```python
from build123d import *

# Parameters (mm, degrees)
BOSS_EXTRUDE1_DEPTH            = 11.43
BOSS_EXTRUDE1_DEPTH_BACK       = 101.6
CUT_EXTRUDE2_REACH             = 833.724
CUT_EXTRUDE2_DIRECTION_2_REACH = 833.724
CUT_EXTRUDE3_REACH             = 833.724
CUT_EXTRUDE3_DIRECTION_2_REACH = 833.724
BOSS_EXTRUDE3_DEPTH            = 149.606
SKETCH9_R                      = 19.05
BOSS_EXTRUDE4_DEPTH            = 101.6
CUT_EXTRUDE4_REACH             = 936.966
CUT_EXTRUDE4_DIRECTION_2_REACH = 936.966
CUT_EXTRUDE5_REACH             = 936.966
CUT_EXTRUDE5_DIRECTION_2_REACH = 936.966


with BuildPart() as part:
    # Sketch1 → Boss-Extrude1 (new, two sides: drawn at the far end of the back side and taken through both)
    with BuildSketch(Plane.XY.offset(-BOSS_EXTRUDE1_DEPTH_BACK)):
        Polygon((-787.4, -209.55), (-787.471663752, -247.65), (-762.071663752, -247.65), (-762.071663752, -209.55), (-203.2, 215.9), (0, 215.9), (0, 241.3), (-203.2, 241.3), (-787.4, -207.01), align=None)
        Polygon((0, 241.3), (0, 215.9), (203.2, 215.9), (762.071663752, -209.55), (762.071663752, -247.65), (787.471663752, -247.65), (787.4, -209.55), (787.4, -207.01), (203.2, 241.3), align=None)
    extrude(amount=BOSS_EXTRUDE1_DEPTH + BOSS_EXTRUDE1_DEPTH_BACK)

    # Sketch5 → Cut-Extrude2 (cut, up to next)
    with BuildSketch(Plane(origin=(0, 0, 0), x_dir=(0, 0, -1), z_dir=(1, 0, 0)), mode=Mode.PRIVATE) as cut_extrude2_sk1:
        Polygon((-11.43, -209.55), (0, 215.9), (0, 241.3), (-11.43, 241.3), (-11.43, 215.9), align=None)
    cut_extrude2_tool1 = extrude(cut_extrude2_sk1.sketch, amount=-CUT_EXTRUDE2_REACH, mode=Mode.PRIVATE) & part.part
    add(cut_extrude2_tool1.solids().sort_by_distance((0, 90.565111, 7.4168))[0], mode=Mode.SUBTRACT)

    # Sketch5 → Cut-Extrude2 direction 2 (cut, up to next)
    with BuildSketch(Plane(origin=(0, 0, 0), x_dir=(0, 0, -1), z_dir=(1, 0, 0)), mode=Mode.PRIVATE) as cut_extrude2_direction_2_sk1:
        Polygon((-11.43, -209.55), (0, 215.9), (0, 241.3), (-11.43, 241.3), (-11.43, 215.9), align=None)
    cut_extrude2_direction_2_tool1 = extrude(cut_extrude2_direction_2_sk1.sketch, amount=CUT_EXTRUDE2_DIRECTION_2_REACH, mode=Mode.PRIVATE) & part.part
    add(cut_extrude2_direction_2_tool1.solids().sort_by_distance((0, 90.565111, 7.4168))[0], mode=Mode.SUBTRACT)

    # Sketch7 → Cut-Extrude3 (cut, up to next)
    with BuildSketch(Plane(origin=(0, 0, 0), x_dir=(0, 0, -1), z_dir=(1, 0, 0)), mode=Mode.PRIVATE) as cut_extrude3_sk1:
        Polygon((26.67, -209.55), (101.6, 223.982414479), (101.6, -247.65), (26.67, -247.65), align=None)
    cut_extrude3_tool1 = extrude(cut_extrude3_sk1.sketch, amount=-CUT_EXTRUDE3_REACH, mode=Mode.PRIVATE) & part.part
    add(cut_extrude3_tool1.solids().sort_by_distance((0, -89.489932, -74.75645))[0], mode=Mode.SUBTRACT)

    # Sketch7 → Cut-Extrude3 direction 2 (cut, up to next)
    with BuildSketch(Plane(origin=(0, 0, 0), x_dir=(0, 0, -1), z_dir=(1, 0, 0)), mode=Mode.PRIVATE) as cut_extrude3_direction_2_sk1:
        Polygon((26.67, -209.55), (101.6, 223.982414479), (101.6, -247.65), (26.67, -247.65), align=None)
    cut_extrude3_direction_2_tool1 = extrude(cut_extrude3_direction_2_sk1.sketch, amount=CUT_EXTRUDE3_DIRECTION_2_REACH, mode=Mode.PRIVATE) & part.part
    add(cut_extrude3_direction_2_tool1.solids().sort_by_distance((0, -89.489932, -74.75645))[0], mode=Mode.SUBTRACT)

    # Sketch8 → Boss-Extrude3 (add)
    with BuildSketch(Plane.XY):
        Polygon((-787.471663752, -247.65), (-762.071663752, -247.65), (-762.071663752, -209.55), (-203.2, 215.9), (203.2, 215.9), (762.071663752, -209.55), (762.071663752, -247.65), (787.471663752, -247.65), (787.4, -207.01), (203.2, 241.3), (-203.2, 241.3), (-787.4, -207.01), align=None)
    extrude(amount=BOSS_EXTRUDE3_DEPTH)

    # Sketch9 → Boss-Extrude4 (add)
    with BuildSketch(Plane(origin=(787.032515479, 1.387837182, 0), x_dir=(0, 0, -1), z_dir=(0.9999984452495948, 0.0017633769855495952, 0))):
        with Locations(Location((-130.556, -229.988224375, 0), (0, 0, 270))):
            Circle(SKETCH9_R)
    boss_extrude4 = extrude(amount=BOSS_EXTRUDE4_DEPTH)

    # Mirror1: Boss-Extrude4 across plane
    add(boss_extrude4.mirror(Plane(origin=(0, 0, 0), x_dir=(0, 0, 1), z_dir=(1, 0, 0))))

    # Cut-Extrude4: up to this face of the body (flat: up to its plane)
    cut_extrude4_end = Plane(part.part.faces().sort_by_distance((-477.863853052, 30.525347549, 40.754880745))[0])
    # Sketch10 → Cut-Extrude4 (cut, up to the picked face)
    with BuildSketch(Plane(origin=(0, 0, 0), x_dir=(0, 0, -1), z_dir=(1, 0, 0)), mode=Mode.PRIVATE) as cut_extrude4_sk1:
        Polygon((-111.506, -207.01), (-111.506, -247.65), (101.6, -247.65), (101.6, 215.9), align=None)
    cut_extrude4_tool1 = split(extrude(cut_extrude4_sk1.sketch, amount=-CUT_EXTRUDE4_REACH, mode=Mode.PRIVATE), bisect_by=cut_extrude4_end, keep=Keep.BOTH, mode=Mode.PRIVATE)
    add(cut_extrude4_tool1.solids().sort_by(Axis((0, -92.041411, -24.838897), (-1, 0, 0)))[0], mode=Mode.SUBTRACT)

    # Cut-Extrude4 direction 2: up to this face of the body (flat: up to its plane)
    cut_extrude4_direction_2_end = Plane(part.part.faces().sort_by_distance((477.863853052, 30.525347549, 40.754880745))[0])
    # Sketch10 → Cut-Extrude4 direction 2 (cut, up to the picked face)
    with BuildSketch(Plane(origin=(0, 0, 0), x_dir=(0, 0, -1), z_dir=(1, 0, 0)), mode=Mode.PRIVATE) as cut_extrude4_direction_2_sk1:
        Polygon((-111.506, -207.01), (-111.506, -247.65), (101.6, -247.65), (101.6, 215.9), align=None)
    cut_extrude4_direction_2_tool1 = split(extrude(cut_extrude4_direction_2_sk1.sketch, amount=CUT_EXTRUDE4_DIRECTION_2_REACH, mode=Mode.PRIVATE), bisect_by=cut_extrude4_direction_2_end, keep=Keep.BOTH, mode=Mode.PRIVATE)
    add(cut_extrude4_direction_2_tool1.solids().sort_by(Axis((0, -92.041411, -24.838897), (1, 0, 0)))[0], mode=Mode.SUBTRACT)

    # Cut-Extrude5: up to this plane
    cut_extrude5_end = Plane(origin=(-191.85340904, 250.007275237, 11.43), z_dir=(-0.6087935435147127, 0.7933286969313537, 0))
    # Sketch11 → Cut-Extrude5 (cut, up to the surface)
    with BuildSketch(Plane(origin=(0, 0, 0), x_dir=(0, 0, -1), z_dir=(1, 0, 0)), mode=Mode.PRIVATE) as cut_extrude5_sk1:
        Polygon((0, 241.3), (-149.606, 241.3), (-149.606, -207.01), (0, 215.9), align=None)
    cut_extrude5_tool1 = split(extrude(cut_extrude5_sk1.sketch, amount=-CUT_EXTRUDE5_REACH, mode=Mode.PRIVATE), bisect_by=cut_extrude5_end, keep=Keep.BOTH, mode=Mode.PRIVATE)
    add(cut_extrude5_tool1.solids().sort_by_distance((0, 91.409357, 97.06341))[0], mode=Mode.SUBTRACT)

    # Cut-Extrude5 direction 2: up to this plane
    cut_extrude5_direction_2_end = Plane(origin=(191.85340904, 250.007275237, 11.43), z_dir=(-0.608793543514713, -0.7933286969313534, 0))
    # Sketch11 → Cut-Extrude5 direction 2 (cut, up to the surface)
    with BuildSketch(Plane(origin=(0, 0, 0), x_dir=(0, 0, -1), z_dir=(1, 0, 0)), mode=Mode.PRIVATE) as cut_extrude5_direction_2_sk1:
        Polygon((0, 241.3), (-149.606, 241.3), (-149.606, -207.01), (0, 215.9), align=None)
    cut_extrude5_direction_2_tool1 = split(extrude(cut_extrude5_direction_2_sk1.sketch, amount=CUT_EXTRUDE5_DIRECTION_2_REACH, mode=Mode.PRIVATE), bisect_by=cut_extrude5_direction_2_end, keep=Keep.BOTH, mode=Mode.PRIVATE)
    add(cut_extrude5_direction_2_tool1.solids().sort_by_distance((0, 91.409357, 97.06341))[0], mode=Mode.SUBTRACT)


solid = part.part
```
Geometry check sheet. Reference: the model listing, model coordinates, mm. A direction names the side the tool comes from. Give positions to 0.01 mm unless a question says otherwise; leave off trailing zeros. Order: outer loops, then holes, each group sorted by start corner. A loop starts at its lowest first (then second) coordinate and runs counter-clockwise, first axis right, second up. Notation, with made-up numbers: (58, 0.25) - (71, 0.25) arc R15 cw to (71, 13.25) - close; hole circle Ø7 at (13, -23). An arc over 180 degrees is marked (long way). Write item = value, one per line. Start each with the question number.
1) Draft check along X on faces 3 (the flat face through (776, -227, 111.506)), 4 (the flat face through (453.4, 49.3, 14.1)), 5 (the flat face through (439.934, 35.683, 33.371)). Enter one of: released by +X, released by -X, zero draft, split by the parting line, or undercut.
2) Section check A-A (y = 184). Enter the section's corners in (x, z), then the cut area to 3 significant figures.
3) Section check B-B (z = 43). Enter the section's corners in (x, y), then the cut area to 3 significant figures.
4) Gauge pin test, flat ends, axial feed: pin 1 Ø14.5 at (x, y) = (779.5, -225) entering from -Z; pin 2 Ø1.5 at (y, z) = (178.5, -25) entering from -X; pin 3 Ø6 at (x, z) = (515.5, 74.5) entering from -Y; pin 4 Ø3 at (x, z) = (95, 3) entering from +Y. Record the tip position at first contact, or that the pin passes through.
5) Access from +Z, -Z, +X, -X, +Y, -Y to the whole of each face (thin tool, end or side, straight path). Record for faces 1 (the flat face through (-442.54, 33.7, 24.12)), 2 (the flat face through (-776, -227, 111.506)).
6) Scan lines: L1, parallel to Y at x = -20, z = -83; L2, parallel to X at y = -58.5, z = 45.5; L3, parallel to X at y = 181.5, z = -77. Record each from-to range of solid material in increasing order.
7) Section check D-D (z = -75.5). Enter the section's corners in (x, y).
8) Section check C-C (x = -29). Enter the section's corners in (y, z), then the cut area to 4 significant figures.
Geometry check:
q1.face_3 = zero draft
q1.face_4 = released by +X
q1.face_5 = undercut
q2.outline = (-277.87, -85.53) - (-245.1, -85.53) - (-245.1, 11.28) - (-277.87, 11.28) - close; (245.1, -85.53) - (277.87, -85.53) - (277.87, 11.28) - (245.1, 11.28) - close
q2.area = 6,340 mm2
q3.outline = (-610.24, -71.06) - (-580.15, -71.06) - (-362.87, 94.35) - (-394.7, 94.35) - close; (362.87, 94.35) - (580.15, -71.06) - (610.24, -71.06) - (394.7, 94.35) - close
q3.area = 10,200 mm2
q4.pin_1 = 111.51
q4.pin_2 = -286.01
q4.pin_3 = -24.13
q4.pin_4 = through
q5.face_1 = +Z, -Z, -Y
q5.face_2 = -Z, +X, -X, -Y
q6.L1 = 215.9 to 241.3
q6.L2 = -593.87 to -563.65, 563.65 to 593.87
q6.L3 = -281.13 to -248.39, 248.39 to 281.13
q7.outline = (-303.79, 164.1) - (-271.24, 164.1) - (-203.2, 215.9) - (203.2, 215.9) - (271.24, 164.1) - (303.79, 164.1) - (203.2, 241.3) - (-203.2, 241.3) - close
q8.outline = (215.9, -100.2) - (223.98, -101.6) - (241.3, -101.6) - (241.3, 0) - (215.9, 0) - close
q8.area = 2,575 mm2
